from build123d import *

# Parameters (mm, degrees)
SKETCH1_W           = 16
SKETCH1_H           = 16
BOSS_EXTRUDE1_DEPTH = 95
SKETCH2_R           = 5
CUT_EXTRUDE1_DEPTH  = 75


with BuildPart() as part:
    # Sketch1 → Boss-Extrude1 (new body)
    with BuildSketch(Plane.XY):
        Rectangle(SKETCH1_W, SKETCH1_H)
    extrude(amount=BOSS_EXTRUDE1_DEPTH)

    # Sketch2 → Cut-Extrude1 (cut)
    with BuildSketch(Plane.ZY.offset(8)):
        with Locations((8, 0)):
            Circle(SKETCH2_R)
    extrude(amount=-CUT_EXTRUDE1_DEPTH, mode=Mode.SUBTRACT)

    # Sketch3 → Revolve1 (revolve)
    with BuildSketch(Plane(origin=(0, 0, 0), x_dir=(0, 0, -1), z_dir=(1, 0, 0))):
        with BuildLine():
            Line((-95, 11.12523004), (-95, 0))
            Line((-95, 0), (-106.12523004, 0))
            ThreePointArc((-106.12523004, 0), (-102.866725603, 7.866725603), (-95, 11.12523004))
        make_face()
    revolve(axis=Axis((0, 0, 95), (0, 0, 1)))


solid = part.part
Source: CAD feature listing. Evaluate the final solid. Frame: model axes, mm. A direction names the side the tool comes from. Coordinates: 2 decimals unless noted, no trailing zeros. Loops run counter-clockwise (first coordinate to the right, second up) from the corner with the lowest first, then second, coordinate; pieces in that order, holes last. Notation, with made-up numbers: (59, 28.25) - (109, 28.25) arc R20 cw to (109, 50.25) - close; hole circle Ø10 at (71.25, 55). An arc over 180 degrees is marked (long way). One line per question, with ' | ' between items.
1) Section D-D, the plane y = 4. Return loops of the section in (x, z), then the cut area to 3 significant figures.
Report:
outline: (-10.38, 95) - (-8, 95) - (-8, 11) - (8, 11) - (8, 95) - (10.38, 95) arc R10.38 ccw to start; (-8, 0) - (8, 0) - (8, 5) - (-8, 5) - close | area: 1,590 mm²
2) Section B-B, the plane z = 8. Return loops of the section in (x, y).
Report:
outline: (-8, -8) - (8, -8) - (8, -5) - (-8, -5) - close; (-8, 5) - (8, 5) - (8, 8) - (-8, 8) - close
3) Line query: line 1 along Y through (x, z) = (2.5, 8); line 2 along X through (y, z) = (4.5, 42.5). Output: solid intervals per line, ascending.
Report:
line 1: y = -8 to -5, 5 to 8 | line 2: x = -8 to 8
4) Set-up query: faces 1 (the face through (0, 8, 47)), 2 (the face through (9, 0, 95)), 3 (the face through (0, -9, 95)), 4 (the face through (-9, 0, 95)), 5 (the face through (0, 0, 0)). Return all of +Z, -Z, +X, -X, +Y, -Y with unobstructed straight access to the full face (end or side cutting, diameter ignored); none if empty.
Report:
face 1: -Z, +X, -X, +Y | face 2: -Z, +X, +Y, -Y | face 3: -Z, +X, -X, -Y | face 4: -Z, -X, +Y, -Y | face 5: -Z, +X, -X, +Y, -Y
5) Section A-A, the plane y = 0. Return loops of the section in (x, z), then the cut area to 3 significant figures.
Report:
outline: (-11.13, 95) - (-8, 95) - (-8, 13) - (8, 13) - (8, 95) - (11.13, 95) arc R11.13 ccw to start; (-8, 0) - (8, 0) - (8, 3) - (-8, 3) - close | area: 1,550 mm²
6) Pull-direction query (Y, two-part tool) for faces 6 (the face through (-0.11, 1.5, 12.77)), 7 (the face through (0, -8, 47)), 8 (the face through (0, 9, 95)); classes: released by +Y, released by -Y, zero draft, split by the parting line, or undercut.
Report:
face 6: undercut | face 7: released by -Y | face 8: zero draft
7) First-contact query: P1, Ø1, axis at x = -5.5, y = -1, coming from the +Z side; P2, Ø13, axis at y = 0, z = 8, coming from the -X side; P3, Ø13, axis at x = 1, z = 47, coming from the +Y side. Flat tips, straight axial feed; report the tip coordinate or a pass-through.
Report:
P1: stops at z = 104.89 | P2: stops at x = -8 | P3: stops at y = 8
8) Section C-C, the plane x = 1.25. Return loops of the section in (y, z), then the cut area to 3 significant figures.
Report:
outline: (-11.05, 95) - (-8, 95) - (-8, 0) - (8, 0) - (8, 95) - (11.05, 95) arc R11.05 ccw to start; hole circle Ø10 at (0, 8) | area: 1,630 mm²
